Design review of the part built by this model. Coordinates are the model's own, in mm. Give positions to 0.01 mm unless a question says otherwise; leave off trailing zeros. Loops run counter-clockwise (first coordinate to the right, second up) from the corner with the lowest first, then second, coordinate; pieces in that order, holes last. Notation, with made-up numbers: (-5, 25.5) -> (6, 25.5) arc R25 cw to (6, 56.5) -> close; hole circle Ø9 at (11.25, 62). An arc over 180 degrees is marked (long way). Answer as CSV lines item,"result".
from build123d import *

# Parameters (mm, degrees)
PAD_DEPTH    = 4
SKETCH001_W  = 0.7
SKETCH001_H  = 0.3
PAD001_DEPTH = 4.6


with BuildPart() as part:
    # Sketch → Pad (new body, symmetric)
    with BuildSketch(Plane.XZ):
        Polygon((-5.3, -5.2), (-5.3, -4.7), (5.3, -4.7), (5.3, -5.2), (5.8, -5.2), (5.8, 5.2), (-5.8, 5.2), (-5.8, -5.2), align=None)
    extrude(amount=PAD_DEPTH, both=True)

    # Sketch001 (on Face2 of Pad) → Pad001 (join)
    with BuildSketch(Plane(origin=(0, 0, -4.7), x_dir=(1, 0, 0), z_dir=(0, 0, -1))):
        with Locations((-2.54, 1.7)):
            Rectangle(SKETCH001_W, SKETCH001_H)
        with Locations((0, 1.7)):
            Rectangle(SKETCH001_W, SKETCH001_H)
        with Locations((2.54, 1.7)):
            Rectangle(SKETCH001_W, SKETCH001_H)
    extrude(amount=PAD001_DEPTH)


solid = part.part
Q1. Clearance check with flat-ended pins moving along their axes: pin 1 Ø0.6 at (x, y) = (5.5, 0.5) entering from -Z; pin 2 Ø2.5 at (x, y) = (-0.5, -1) entering from -Z; pin 3 Ø0.8 at (x, z) = (-2.5, -6.5) entering from -Y; pin 4 Ø0.6 at (x, z) = (-2.5, -8) entering from +Y. State where each tip first meets the part, or that it passes through.
Filled sheet:
pin 1,"stops at z = -5.2"
pin 2,"stops at z = -9.3"
pin 3,"stops at y = -1.85"
pin 4,"stops at y = -1.55"
Q2. The part is to be moulded in two halves that separate along X. For faces 1 (the flat face through (-5.8, 0, 0)), 2 (the flat face through (0, 0, -4.7)), 3 (the flat face through (5.8, 0, 0)), 4 (the flat face through (0, 0, 5.2)), say which applies: pulls with the +X half, pulls with the -X half, needs draft (parallel to the pull), parting line crosses it, or undercut.
Filled sheet:
face 1,"pulls with the -X half"
face 2,"undercut"
face 3,"pulls with the +X half"
face 4,"needs draft"
Q3. We need section A-A, the plane z = -7. State the section outline as (x, y) points.
Filled sheet:
outline,"(-2.89, -1.85) -> (-2.19, -1.85) -> (-2.19, -1.55) -> (-2.89, -1.55) -> close; (-0.35, -1.85) -> (0.35, -1.85) -> (0.35, -1.55) -> (-0.35, -1.55) -> close; (2.19, -1.85) -> (2.89, -1.85) -> (2.89, -1.55) -> (2.19, -1.55) -> close"
Q4. We need section D-D, the plane x = 4. State the section outline as (y, z) points.
Filled sheet:
outline,"(-4, -4.7) -> (4, -4.7) -> (4, 5.2) -> (-4, 5.2) -> close"
Q5. We need section B-B, the plane z = -5. State the section outline as (x, y) points.
Filled sheet:
outline,"(-5.8, -4) -> (-5.3, -4) -> (-5.3, 4) -> (-5.8, 4) -> close; (-2.89, -1.85) -> (-2.19, -1.85) -> (-2.19, -1.55) -> (-2.89, -1.55) -> close; (-0.35, -1.85) -> (0.35, -1.85) -> (0.35, -1.55) -> (-0.35, -1.55) -> close; (2.19, -1.85) -> (2.89, -1.85) -> (2.89, -1.55) -> (2.19, -1.55) -> close; (5.3, -4) -> (5.8, -4) -> (5.8, 4) -> (5.3, 4) -> close"
Q6. We need section C-C, the plane y = -0.75. State the section outline as (x, z) points.
Filled sheet:
outline,"(-5.8, -5.2) -> (-5.3, -5.2) -> (-5.3, -4.7) -> (5.3, -4.7) -> (5.3, -5.2) -> (5.8, -5.2) -> (5.8, 5.2) -> (-5.8, 5.2) -> close"
Q7. To check wall thickness, follow probe 1 along X at (y, z) = (1.75, -4.75); probe 2 along Z at (x, y) = (4.25, 1.5); probe 3 along Y at (x, z) = (0, -6.75). State the ranges of each line that lie inside material, in increasing order. Write a range as from..to.
Filled sheet:
probe 1,"x = -5.8..-5.3, 5.3..5.8"
probe 2,"z = -4.7..5.2"
probe 3,"y = -1.85..-1.55"
